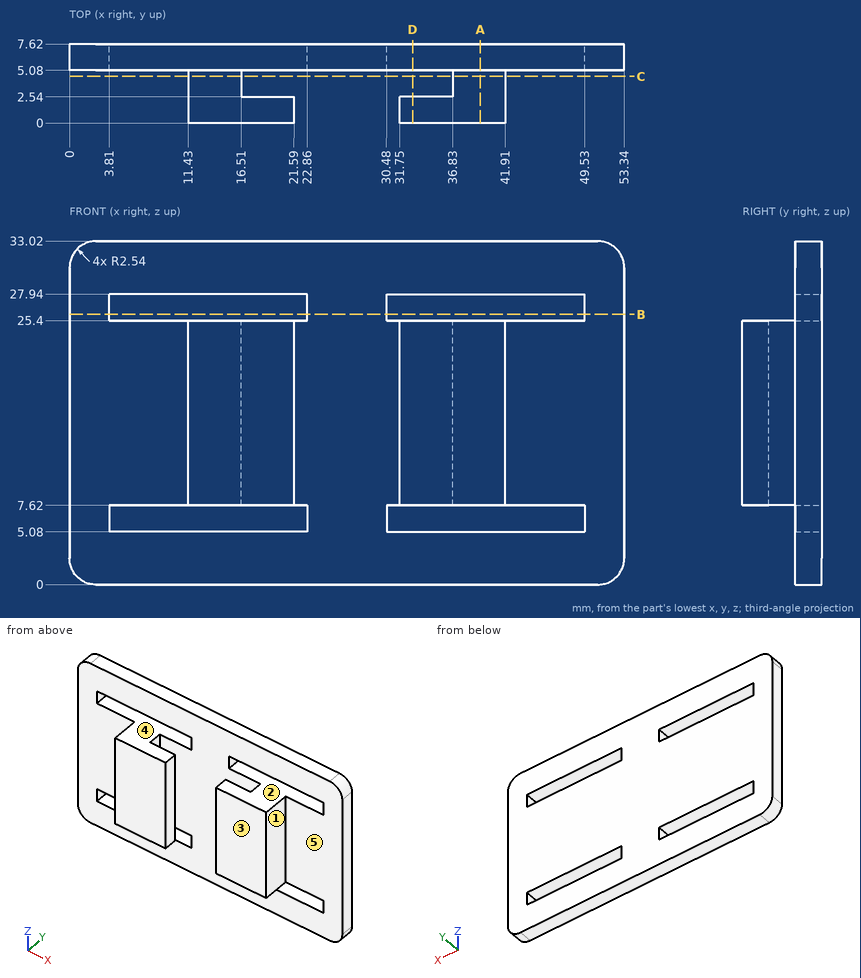
Study the drawing (mm; zero at the part's minimum x, y, z) and answer. A direction names the side the tool comes from. Coordinates: 2 decimals unless noted, no trailing zeros. Loops run counter-clockwise (first coordinate to the right, second up) from the corner with the lowest first, then second, coordinate; pieces in that order, holes last. Notation, with made-up numbers: (85, -9.75) -> (116, -9.75) arc R24 ccw to (116, 25.25) -> close; hole circle Ø5 at (11.5, -35.5). An arc over 180 degrees is marked (long way). Answer as CSV lines item,"result".
1) Flat-ended cylindrical pins translate along their axes: pin 1 (10 mm diameter, centred on x = 30.5, z = 9.5, fed in from -Y); pin 2 (3 mm diameter, centred on x = 15.5, y = 2.5, fed in from -Z); pin 3 (3 mm diameter, centred on y = 1, z = 15, fed in from -X); pin 4 (1.3 mm diameter, centred on y = 3.5, z = 17.5, fed in from +X). Find the tip coordinate at first contact, or state that the pin passes through.
A:
pin 1,"stops at y = 0"
pin 2,"stops at z = 7.62"
pin 3,"stops at x = 11.43"
pin 4,"stops at x = 41.91"
2) For the marked faces 1, 2 and 3, determine the directions among +Z, -Z, +X, -X, +Y, -Y from which every point of the face is accessible in a straight line to the end or side of a thin tool.
A:
face 1,"+Z, -Z, +X, -Y"
face 2,"+Y, -Y"
face 3,"+Z, -Z, +X, -X, -Y"
3) The part is cut by section B-B (z = 26). Give the vertices of the cut face in (x, y).
A:
outline,"(0, 5.08) -> (3.81, 5.08) -> (3.81, 7.62) -> (0, 7.62) -> close; (22.86, 5.08) -> (30.48, 5.08) -> (30.48, 7.62) -> (22.86, 7.62) -> close; (49.53, 5.08) -> (53.34, 5.08) -> (53.34, 7.62) -> (49.53, 7.62) -> close"
4) For a pull along Z with two mould halves and no side action, classify the marked faces 4 and 5 as released by +Z, released by -Z, zero draft, split by the parting line, or undercut.
A:
face 4,"undercut"
face 5,"zero draft"
5) The part is cut by section D-D (x = 33). Give the vertices of the cut face in (y, z).
A:
outline,"(0, 7.62) -> (2.54, 7.62) -> (2.54, 25.4) -> (0, 25.4) -> close; (5.08, 0) -> (7.62, 0) -> (7.62, 5.08) -> (5.08, 5.08) -> close; (5.08, 7.62) -> (7.62, 7.62) -> (7.62, 25.4) -> (5.08, 25.4) -> close; (5.08, 27.94) -> (7.62, 27.94) -> (7.62, 33.02) -> (5.08, 33.02) -> close"
6) The part is cut by section C-C (y = 4.5). Give the vertices of the cut face in (x, z).
A:
outline,"(11.43, 7.62) -> (16.51, 7.62) -> (16.51, 25.4) -> (11.43, 25.4) -> close; (36.83, 7.62) -> (41.91, 7.62) -> (41.91, 25.4) -> (36.83, 25.4) -> close"
7) Straight lines are drawn through the part: probe 1 along Z at (x, y) = (13.5, 6.75); probe 2 along X at (y, z) = (6, 6); probe 3 along Y at (x, z) = (32, 18). For each, find the intervals that lie inside material, in ascending order.
A:
probe 1,"z = 0 to 5.08, 7.62 to 25.4, 27.94 to 33.02"
probe 2,"x = 0 to 3.81, 22.86 to 30.48, 49.53 to 53.34"
probe 3,"y = 0 to 2.54, 5.08 to 7.62"
8) The part is cut by section A-A (x = 39.5). Give the vertices of the cut face in (y, z), and give its area (3 significant figures).
A:
outline,"(0, 7.62) -> (7.62, 7.62) -> (7.62, 25.4) -> (0, 25.4) -> close; (5.08, 0) -> (7.62, 0) -> (7.62, 5.08) -> (5.08, 5.08) -> close; (5.08, 27.94) -> (7.62, 27.94) -> (7.62, 33.02) -> (5.08, 33.02) -> close"
area,"161 mm²"
